Input: part model. Units: mm. Frame: model coordinates. Round coordinates to 2 decimals unless told otherwise and drop trailing zeros. Loops run counter-clockwise (first coordinate to the right, second up) from the corner with the lowest first, then second, coordinate; pieces in that order, holes last. Notation, with made-up numbers: (62.25, -8.75) - (119.25, -8.75) arc R34 ccw to (119.25, 22.25) - close; hole circle Ø6 at (68, -18.75). An arc over 180 degrees is marked (long way). Use CSV: the item, a comma, the result in double quotes. Start each with the question number.
1. Pin query (flat end, axial travel): P1, Ø10, axis at y = -10, z = -33.5, coming from the +X side; P2, Ø1, axis at y = -8.5, z = 7.5, coming from the -X side; P3, Ø2, axis at x = 44, y = -0.5, coming from the -Z side. Return the tip coordinate at first contact, or that it passes through.
2. Cut plane C-C (x = -53.5). Return loops of the section in (y, z), and give its area (3 significant figures).
3. Cut plane A-A (y = -18). Return loops of the section in (x, z).
4. Material intervals for probe 1 along X at (y, z) = (-15, 17.5); probe 2 along Z at (x, y) = (-22, -25.5); probe 3 along Z at (x, y) = (4, 34), sorted ascending. Write a range as from..to.
5. Cut plane B-B (z = -12). Return loops of the section in (x, y), and give its area (3 significant figures).
6. Cut plane D-D (y = 17). Return loops of the section in (x, z), and give its area (3 significant figures).
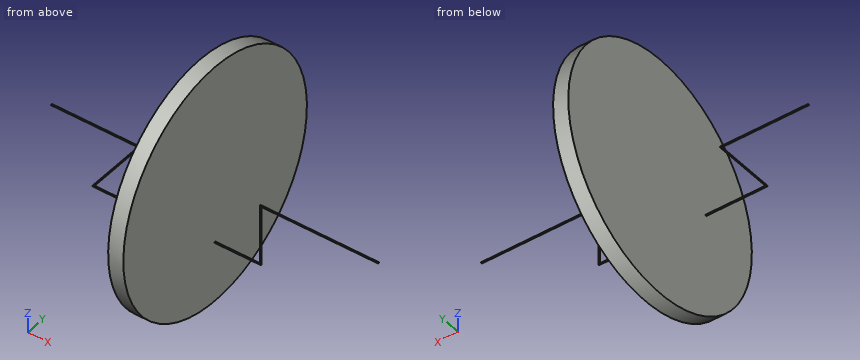
```python
from build123d import *

# Parameters (mm, degrees)
F0_W = 6.35
F0_H = 50.8
F4_R = 0.254
F8_R = 0.254


with BuildPart() as f1:
    # F0 (on Front) → F1 (revolve)
    with BuildSketch(Plane.XZ):
        with Locations((3.175, 25.4)):
            Rectangle(F0_W, F0_H)
    revolve(axis=Axis((3.175, 0, 0), (1, 0, 0)))

    # F5: sweep along a path in F2
    with BuildLine(Plane.XY) as f5_path:
        Line((0, -25.4), (-25.4, -25.4))
        Line((-25.4, -25.4), (-25.4, 0))
        Line((-25.4, 0), (-62.0676704339, 0))
    # F4 (on offset) → F5 (sweep)
    with BuildSketch(Plane.YZ.offset(-33.02)):
        Circle(F4_R)
    sweep(path=f5_path.line, transition=Transition.RIGHT)

    # F9: sweep along a path in F6
    with BuildLine(Plane.XZ) as f9_path:
        Line((74.6657835295, 0), (25.4, 0))
        Line((25.4, 0), (25.4, -25.4))
        Line((25.4, -25.4), (0, -25.4))
    # F8 (on offset) → F9 (sweep)
    with BuildSketch(Plane.YZ.offset(33.02)):
        Circle(F8_R)
    sweep(path=f9_path.line, transition=Transition.RIGHT)


solid = f1.part
```
Established:
1,P1,"stops at x = 6.35"
1,P2,"stops at x = 0"
1,P3,"stops at z = -0.25"
2,outline,"circle Ø0.51 at (0, 0)"
2,area,"0.203 mm2"
3,outline,"circle Ø0.51 at (-25.4, 0); (0, -47.5) - (6.35, -47.5) - (6.35, 47.5) - (0, 47.5) - close"
4,probe 1,"x = 0..6.35"
4,probe 2,"z = -0.23..0.23"
4,probe 3,"z = -37.74..37.74"
5,outline,"(0, -49.36) - (6.35, -49.36) - (6.35, 49.36) - (0, 49.36) - close; circle Ø0.51 at (25.4, 0)"
5,area,"627 mm2"
6,outline,"(0, -47.87) - (6.35, -47.87) - (6.35, 47.87) - (0, 47.87) - close"
6,area,"608 mm2"
